Read the model definition and answer for the solid it produces. Units are mm, in the model's axes. A direction names the side the tool comes from. Coordinates: 2 decimals unless noted, no trailing zeros. Write each loop counter-clockwise with the first axis right and the second up, starting at its lowest first coordinate (ties: lowest second). Pieces come first, ordered by that corner, then holes.
Item 1: Each of these flat-tipped pins is pushed along its axis until it touches: P1, Ø3, axis at x = 10.5, y = 8.5, coming from the +Z side; P2, Ø1, axis at x = 14.5, y = 19, coming from the -Z side; P3, Ø7.5, axis at x = 12, y = 19.5, coming from the +Z side; P4, Ø3.5, axis at y = -10.86, z = 67.5, coming from the -X side. Where does it stop, or does it pass through?
Item 2: Determine the mould class of faces 1 (the face through (13.832, 1.637, -22.827)), 2 (the face through (25.9, 0, -95)), 3 (the face through (14, 22, -75)) for opening direction X: released by +X, released by -X, zero draft, split by the parting line, or undercut.
Item 3: Section A-A (y = 18) is taken. Give the vertices of the cut face in (x, z).
Item 4: Section B-B (z = 51) is taken. Give the vertices of the cut face in (x, y).
Item 5: Straight lines are drawn through the part: probe 1 along Z at (x, y) = (22.75, 25); probe 2 along Z at (x, y) = (13.75, -12); probe 3 along Z at (x, y) = (11.75, 21). For each, find the intervals that lie inside material, in ascending order.
Item 6: A tool of negligible diameter and unlimited length cuts with its end or side. For faces 4 (the face through (14, 22, -15)), 5 (the face through (14, 14.5, 98)), 6 (the face through (26, 23, 60)), 7 (the face through (2.958, -0.931, 152.957)), from which of +Z, -Z, +X, -X, +Y, -Y can it reach the whole face along a straight path? Write none if from no direction.
from build123d import *

# Parameters (mm, degrees)
SKETCH_1_W           = 250
SKETCH_1_H           = 29
SKETCH_1_W_2         = 30
SKETCH_1_H_2         = 15
EXTRUDE_1_DEPTH      = 28
SKETCH_1_3_R         = 2
CUT_EXTRUDE_1_DEPTH  = 132.450561049
CUT_EXTRUDE_START    = 2
SKETCH_1_5_R         = 2
CUT_EXTRUDE_2_DEPTH  = 24
SKETCH_3_W           = 6
SKETCH_3_H           = 19
EXTRUDE_2_DEPTH      = 35
SKETCH_3_3_W         = 6
SKETCH_3_3_H         = 19
EXTRUDE_3_DEPTH      = 35
SKETCH_1_6_R         = 2
CUT_EXTRUDE_3_DEPTH  = 166.088612569
CUT_EXTRUDE_7_REACH  = 167.089
SKETCH_1_8_R         = 3.1
FILLET_1_R           = 9.5
FILLET_2_R           = 5
SKETCH_4_R           = 5.1
CUT_EXTRUDE_4_DEPTH  = 31.5
SKETCH_4_2_OUTSIDE_W = 87.946
SKETCH_4_2_OUTSIDE_H = 103.946
SKETCH_4_2_OUTSIDE_R = 5.1
CUT_EXTRUDE_5_DEPTH  = 21.5
SKETCH_5_OUTSIDE_W   = 83.722
SKETCH_5_OUTSIDE_H   = 99.722
SKETCH_5_OUTSIDE_W_2 = 23.8
SKETCH_5_OUTSIDE_H_2 = 24.8
CUT_EXTRUDE_6_DEPTH  = 18


with BuildPart() as part:
    # 草图1 → 凸台-拉伸1 (new body)
    with BuildSketch(Plane(origin=(0, 0, 0), x_dir=(0, 0, -1), z_dir=(1, 0, 0))):
        Rectangle(SKETCH_1_W, SKETCH_1_H)
        with Locations((-60, 22)):
            Rectangle(SKETCH_1_W_2, SKETCH_1_H_2)
        with Locations((0, 22)):
            Rectangle(SKETCH_1_W_2, SKETCH_1_H_2)
        with Locations((60, 22)):
            Rectangle(SKETCH_1_W_2, SKETCH_1_H_2)
    extrude(amount=EXTRUDE_1_DEPTH)

    # 草图1<3> → 切除-拉伸1 (cut, through all)
    with BuildSketch(Plane(origin=(0, 0, 0), x_dir=(0, 0, -1), z_dir=(1, 0, 0))):
        with Locations((-67.5, -10.858617882)):
            Circle(SKETCH_1_3_R)
        with Locations((-22.5, -10.858617882)):
            Circle(SKETCH_1_3_R)
        with Locations((22.5, -10.858617882)):
            Circle(SKETCH_1_3_R)
        with Locations((-60, 25.5)):
            Circle(SKETCH_1_3_R)
        with Locations((67.5, -10.858617882)):
            Circle(SKETCH_1_3_R)
        with Locations((0, 25.5)):
            Circle(SKETCH_1_3_R)
        with Locations((60, 25.5)):
            Circle(SKETCH_1_3_R)
    extrude(amount=CUT_EXTRUDE_1_DEPTH, mode=Mode.SUBTRACT)

    # 草图1<5> → 切除-拉伸2 (cut)
    # profile 1 of 7: a face of its own
    with BuildSketch(Plane(origin=(0, 0, 0), x_dir=(0, 0, -1), z_dir=(1, 0, 0)).offset(CUT_EXTRUDE_START)):
        with BuildLine():
            Line((-72.5, 29.5), (-72.5, 25.5))
            ThreePointArc((-72.5, 25.5), (-60, 13), (-47.5, 25.5))
            Line((-47.5, 25.5), (-47.5, 29.5))
            Line((-47.5, 29.5), (-72.5, 29.5))
        make_face()
        with Locations((-60, 25.5)):
            Circle(SKETCH_1_5_R, mode=Mode.SUBTRACT)
    # profile 2 of 7: a face of its own
    with BuildSketch(Plane(origin=(0, 0, 0), x_dir=(0, 0, -1), z_dir=(1, 0, 0)).offset(CUT_EXTRUDE_START)):
        with BuildLine():
            Line((-79.457856675, -14.5), (-55.542143325, -14.5))
            ThreePointArc((-55.542143325, -14.5), (-67.5, 1.641382118), (-79.457856675, -14.5))
        make_face()
        with Locations((-67.5, -10.858617882)):
            Circle(SKETCH_1_5_R, mode=Mode.SUBTRACT)
    # profile 3 of 7: a face of its own
    with BuildSketch(Plane(origin=(0, 0, 0), x_dir=(0, 0, -1), z_dir=(1, 0, 0)).offset(CUT_EXTRUDE_START)):
        with BuildLine():
            Line((-34.457856675, -14.5), (-10.542143325, -14.5))
            ThreePointArc((-10.542143325, -14.5), (-22.5, 1.641382118), (-34.457856675, -14.5))
        make_face()
        with Locations((-22.5, -10.858617882)):
            Circle(SKETCH_1_5_R, mode=Mode.SUBTRACT)
    # profile 4 of 7: a face of its own
    with BuildSketch(Plane(origin=(0, 0, 0), x_dir=(0, 0, -1), z_dir=(1, 0, 0)).offset(CUT_EXTRUDE_START)):
        with BuildLine():
            ThreePointArc((-12.5, 25.5), (0, 13), (12.5, 25.5))
            Line((12.5, 25.5), (12.5, 29.5))
            Line((12.5, 29.5), (-12.5, 29.5))
            Line((-12.5, 29.5), (-12.5, 25.5))
        make_face()
        with Locations((0, 25.5)):
            Circle(SKETCH_1_5_R, mode=Mode.SUBTRACT)
    # profile 5 of 7: a face of its own
    with BuildSketch(Plane(origin=(0, 0, 0), x_dir=(0, 0, -1), z_dir=(1, 0, 0)).offset(CUT_EXTRUDE_START)):
        with BuildLine():
            Line((10.542143325, -14.5), (34.457856675, -14.5))
            ThreePointArc((34.457856675, -14.5), (22.5, 1.641382118), (10.542143325, -14.5))
        make_face()
        with Locations((22.5, -10.858617882)):
            Circle(SKETCH_1_5_R, mode=Mode.SUBTRACT)
    # profile 6 of 7: a face of its own
    with BuildSketch(Plane(origin=(0, 0, 0), x_dir=(0, 0, -1), z_dir=(1, 0, 0)).offset(CUT_EXTRUDE_START)):
        with BuildLine():
            Line((55.542143325, -14.5), (79.457856675, -14.5))
            ThreePointArc((79.457856675, -14.5), (67.5, 1.641382118), (55.542143325, -14.5))
        make_face()
        with Locations((67.5, -10.858617882)):
            Circle(SKETCH_1_5_R, mode=Mode.SUBTRACT)
    # profile 7 of 7: a face of its own
    with BuildSketch(Plane(origin=(0, 0, 0), x_dir=(0, 0, -1), z_dir=(1, 0, 0)).offset(CUT_EXTRUDE_START)):
        with BuildLine():
            ThreePointArc((47.5, 25.5), (60, 13), (72.5, 25.5))
            Line((72.5, 25.5), (72.5, 29.5))
            Line((72.5, 29.5), (47.5, 29.5))
            Line((47.5, 29.5), (47.5, 25.5))
        make_face()
        with Locations((60, 25.5)):
            Circle(SKETCH_1_5_R, mode=Mode.SUBTRACT)
    extrude(amount=CUT_EXTRUDE_2_DEPTH, mode=Mode.SUBTRACT)

    # 草图3 → 凸台-拉伸2 (add)
    with BuildSketch(Plane.XY.offset(125)):
        with Locations((25, 0)):
            Rectangle(SKETCH_3_W, SKETCH_3_H)
    extrude(amount=EXTRUDE_2_DEPTH)

    # 草图3<3> → 凸台-拉伸3 (add)
    with BuildSketch(Plane.XY.offset(125)):
        with Locations((25, 0)):
            Rectangle(SKETCH_3_3_W, SKETCH_3_3_H)
        with Locations((3, 0)):
            Rectangle(SKETCH_3_3_W, SKETCH_3_3_H)
    extrude(amount=EXTRUDE_3_DEPTH)

    # 草图1<6> → 切除-拉伸3 (cut, through all)
    with BuildSketch(Plane(origin=(0, 0, 0), x_dir=(0, 0, -1), z_dir=(1, 0, 0))):
        with Locations(Location((-150, 0, 0), (0, 0, 90))):
            Circle(SKETCH_1_6_R)
    extrude(amount=CUT_EXTRUDE_3_DEPTH, mode=Mode.SUBTRACT)

    # 草图1<8> → 切除-拉伸7 (cut, up to next)
    with BuildSketch(Plane(origin=(0, 0, 0), x_dir=(0, 0, -1), z_dir=(1, 0, 0)), mode=Mode.PRIVATE) as cut_extrude_7_sk1:
        with Locations(Location((-150, 0, 0), (0, 0, 180))):
            Circle(SKETCH_1_8_R)
    cut_extrude_7_tool1 = extrude(cut_extrude_7_sk1.sketch, amount=CUT_EXTRUDE_7_REACH, mode=Mode.PRIVATE) & part.part
    add(cut_extrude_7_tool1.solids().sort_by_distance((0, 0, 150))[0], mode=Mode.SUBTRACT)

    # 圆角1
    fillet_1_edges = [part.edges().sort_by_distance(p)[0] for p in [
        (25, 9.5, 160),
        (25, -9.5, 160),
        (3, -9.5, 160),
        (3, 9.5, 160),
    ]]
    fillet(fillet_1_edges, radius=FILLET_1_R - 0.0001)  # a hair under: the kernel refuses the full size

    # 圆角2
    fillet_2_edges = [part.edges().sort_by_distance(p)[0] for p in [
        (14, -14.5, 125),
        (14, 14.5, 125),
    ]]
    fillet(fillet_2_edges, radius=FILLET_2_R)

    # 草图4 → 切除-拉伸4 (cut)
    with BuildSketch(Plane(origin=(0, 0, -125), x_dir=(-1, 0, 0), z_dir=(0, 0, -1))):
        with Locations((-14, 0)):
            Circle(SKETCH_4_R)
    extrude(amount=-CUT_EXTRUDE_4_DEPTH, mode=Mode.SUBTRACT)

    # 草图4<2> outside → 切除-拉伸5 (cut)
    with BuildSketch(Plane(origin=(0, 0, -125), x_dir=(-1, 0, 0), z_dir=(0, 0, -1))):
        with Locations((-14, 7.5)):
            Rectangle(SKETCH_4_2_OUTSIDE_W, SKETCH_4_2_OUTSIDE_H)
        with Locations((-14, 0)):
            Circle(SKETCH_4_2_OUTSIDE_R, mode=Mode.SUBTRACT)
    extrude(amount=-CUT_EXTRUDE_5_DEPTH, mode=Mode.SUBTRACT)

    # 草图5 outside → 切除-拉伸6 (cut)
    with BuildSketch(Plane(origin=(0, 0, -103.5), x_dir=(-1, 0, 0), z_dir=(0, 0, -1))):
        with Locations((-14, 7.5)):
            Rectangle(SKETCH_5_OUTSIDE_W, SKETCH_5_OUTSIDE_H)
        with Locations((-14, 0)):
            Rectangle(SKETCH_5_OUTSIDE_W_2, SKETCH_5_OUTSIDE_H_2, mode=Mode.SUBTRACT)
    extrude(amount=-CUT_EXTRUDE_6_DEPTH, mode=Mode.SUBTRACT)


solid = part.part
Established:
1. P1: stops at z = 125
1. P2: stops at z = -75
1. P3: stops at z = 75
1. P4: passes through
2. face 1: undercut
2. face 2: released by +X
2. face 3: zero draft
3. outline: (0, -75) - (28, -75) - (28, -45) - (0, -45) - close; (0, -15) - (28, -15) - (28, 15) - (0, 15) - close; (0, 45) - (28, 45) - (28, 75) - (0, 75) - close; hole (2, -70) - (26, -70) - (26, -50) - (2, -50) - close; hole (2, -10) - (26, -10) - (26, 10) - (2, 10) - close; hole (2, 50) - (26, 50) - (26, 70) - (2, 70) - close
4. outline: (0, -14.5) - (28, -14.5) - (28, 29.5) - (26, 29.5) - (26, 16.83) - (2, 16.83) - (2, 29.5) - (0, 29.5) - close
5. probe 1: z = -75 to -72.49, -47.51 to -45, -15 to -12.49, 12.49 to 15, 45 to 47.51, 72.49 to 75
5. probe 2: z = -103.5 to -79.95, -55.05 to -34.95, -10.05 to 10.05, 34.95 to 55.05, 79.95 to 124.33
5. probe 3: z = -75 to -71.66, -48.34 to -45, -15 to -11.66, 11.66 to 15, 45 to 48.34, 71.66 to 75
6. face 4: +X, -X, +Y
6. face 5: +Z, +X, -X, +Y
6. face 6: +Y
6. face 7: -X
